Geometry: final body of the model. Coordinates: model frame, mm. Face numbers are marked on the shaded views. Give positions to 0.01 mm unless a question says otherwise; leave off trailing zeros. Write each loop counter-clockwise with the first axis right and the second up, starting at its lowest first coordinate (ties: lowest second). Pieces come first, ordered by that corner, then holes. Notation, with made-up numbers: (25, 35) -> (48, 35) arc R38 ccw to (48, 74) -> close; hole circle Ø10 at (-8.75, 30.25). An arc over 180 degrees is marked (long way). Answer as a JSON object with one key per item and string values.
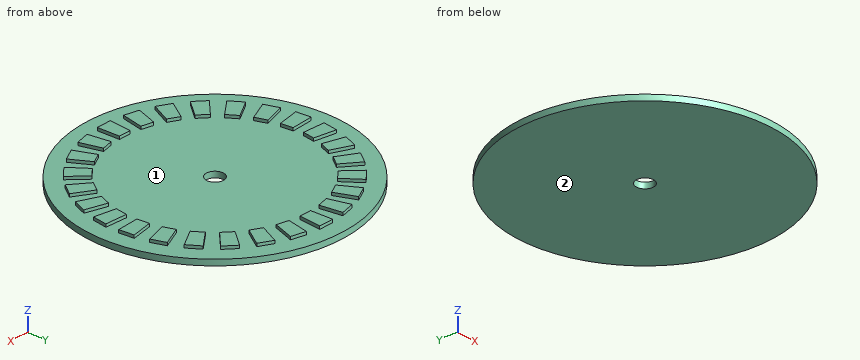
from build123d import *

# Parameters (mm, degrees)
SKETCH1_R           = 45
SKETCH1_R_2         = 3
BOSS_EXTRUDE1_DEPTH = 2
BOSS_EXTRUDE2_DEPTH = 1


with BuildPart() as part:
    # Sketch1 → Boss-Extrude1 (new body)
    with BuildSketch(Plane.XY):
        Circle(SKETCH1_R)
        Circle(SKETCH1_R_2, mode=Mode.SUBTRACT)
    extrude(amount=BOSS_EXTRUDE1_DEPTH)

    # Sketch2 → Boss-Extrude2 (add)
    with BuildSketch(Plane.XY.offset(2)):
        Polygon((2.5, 39.592009569), (-2.5, 39.592009569), (-2.028723843, 32.128501517), (2.028723843, 32.128501517), align=None)
        Polygon((11.902342614, 37.843248566), (7.047633527, 39.039826887), (5.719080868, 31.680411048), (9.658626498, 30.70940026), align=None)
        Polygon((20.612964339, 33.895175511), (16.18568421, 36.218791371), (13.134513387, 29.391170243), (16.727204889, 27.505580284), align=None)
        Polygon((28.125635501, 27.977238059), (24.38308176, 31.29285135), (19.78661573, 25.393821456), (22.823658933, 22.703235961), align=None)
        Polygon((34.003746961, 20.433365224), (31.163423227, 24.548284553), (25.288791888, 19.920676068), (27.59368488, 16.581462086), align=None)
        Polygon((37.905684245, 11.701979474), (36.13265981, 16.377060688), (29.321275383, 13.289813396), (30.760066161, 9.496033907), align=None)
        Polygon((39.604680943, 2.290517213), (39.001997542, 7.254061583), (31.64971293, 5.886595076), (32.138784205, 1.858730753), align=None)
        Polygon((39.001997542, -7.254061583), (39.604680943, -2.290517213), (32.138784205, -1.858730753), (31.64971293, -5.886595076), align=None)
        Polygon((36.13265981, -16.377060688), (37.905684245, -11.701979474), (30.760066161, -9.496033907), (29.321275383, -13.289813396), align=None)
        Polygon((31.163423227, -24.548284553), (34.003746961, -20.433365224), (27.59368488, -16.581462086), (25.288791888, -19.920676068), align=None)
        Polygon((24.38308176, -31.29285135), (28.125635501, -27.977238059), (22.823658933, -22.703235961), (19.78661573, -25.393821456), align=None)
        Polygon((16.18568421, -36.218791371), (20.612964339, -33.895175511), (16.727204889, -27.505580284), (13.134513387, -29.391170243), align=None)
        Polygon((7.047633527, -39.039826887), (11.902342614, -37.843248566), (9.658626498, -30.70940026), (5.719080868, -31.680411048), align=None)
        Polygon((-2.5, -39.592009569), (2.5, -39.592009569), (2.028723843, -32.128501517), (-2.028723843, -32.128501517), align=None)
        Polygon((-11.902342614, -37.843248566), (-7.047633527, -39.039826887), (-5.719080868, -31.680411048), (-9.658626498, -30.70940026), align=None)
        Polygon((-20.612964339, -33.895175511), (-16.18568421, -36.218791371), (-13.134513387, -29.391170243), (-16.727204889, -27.505580284), align=None)
        Polygon((-28.125635501, -27.977238059), (-24.38308176, -31.29285135), (-19.78661573, -25.393821456), (-22.823658933, -22.703235961), align=None)
        Polygon((-34.003746961, -20.433365224), (-31.163423227, -24.548284553), (-25.288791888, -19.920676068), (-27.59368488, -16.581462086), align=None)
        Polygon((-37.905684245, -11.701979474), (-36.13265981, -16.377060688), (-29.321275383, -13.289813396), (-30.760066161, -9.496033907), align=None)
        Polygon((-39.604680943, -2.290517213), (-39.001997542, -7.254061583), (-31.64971293, -5.886595076), (-32.138784205, -1.858730753), align=None)
        Polygon((-39.001997542, 7.254061583), (-39.604680943, 2.290517213), (-32.138784205, 1.858730753), (-31.64971293, 5.886595076), align=None)
        Polygon((-36.13265981, 16.377060688), (-37.905684245, 11.701979474), (-30.760066161, 9.496033907), (-29.321275383, 13.289813396), align=None)
        Polygon((-31.163423227, 24.548284553), (-34.003746961, 20.433365224), (-27.59368488, 16.581462086), (-25.288791888, 19.920676068), align=None)
        Polygon((-24.38308176, 31.29285135), (-28.125635501, 27.977238059), (-22.823658933, 22.703235961), (-19.78661573, 25.393821456), align=None)
        Polygon((-16.18568421, 36.218791371), (-20.612964339, 33.895175511), (-16.727204889, 27.505580284), (-13.134513387, 29.391170243), align=None)
        Polygon((-7.047633527, 39.039826887), (-11.902342614, 37.843248566), (-9.658626498, 30.70940026), (-5.719080868, 31.680411048), align=None)
    extrude(amount=BOSS_EXTRUDE2_DEPTH)


solid = part.part
Q1. Cut plane A-A (x = 0). Return the cut outline in (y, z), and give its area (3 significant figures).
Values:
{"outline": "(-45, 0) -> (-3, 0) -> (-3, 2) -> (-32.13, 2) -> (-32.13, 3) -> (-39.59, 3) -> (-39.59, 2) -> (-45, 2) -> close; (3, 0) -> (45, 0) -> (45, 2) -> (39.59, 2) -> (39.59, 3) -> (32.13, 3) -> (32.13, 2) -> (3, 2) -> close", "area": "183 mm²"}
Q2. Cut plane C-C (z = 2.45). State how many separate pieces and enclosed holes the cut face has, and give its area (3 significant figures).
Values:
{"separate pieces": "26", "enclosed holes": "0", "area": "879 mm²"}
Q3. First-contact query: P1, Ø4, axis at x = -21.5, y = -12, coming from the +Z side; P2, Ø0.5, axis at x = 1, z = 2.5, coming from the +Y side; P3, Ø0.5, axis at x = -1, z = 2.5, coming from the -Y side. Flat tips, straight axial feed; report the tip coordinate or a pass-through.
Values:
{"P1": "z = 2", "P2": "y = 39.59", "P3": "y = -39.59"}
Q4. Material intervals for L1, parallel to Y at x = 0, z = 1.15; L2, parallel to X at y = 37, z = 2.5; L3, parallel to Z at x = 31.5, y = -16, sorted ascending. Write a range as from..to.
Values:
{"L1": "-45..-3, 3..45", "L2": "-11.64..-6.68, -2.34..2.34, 6.68..11.64", "L3": "0..2"}
Q5. Cut plane B-B (y = 0). Return the cut outline in (x, z).
Values:
{"outline": "(-45, 0) -> (-3, 0) -> (-3, 2) -> (-45, 2) -> close; (3, 0) -> (45, 0) -> (45, 2) -> (3, 2) -> close"}
Q6. Mould query, pull axis Y, two halves, no side actions, for the marked faces 1 and 2. Classes: pulls with the +Y half, pulls with the -Y half, needs draft (parallel to the pull), parting line crosses it, or undercut.
Values:
{"face 1": "undercut", "face 2": "needs draft"}
